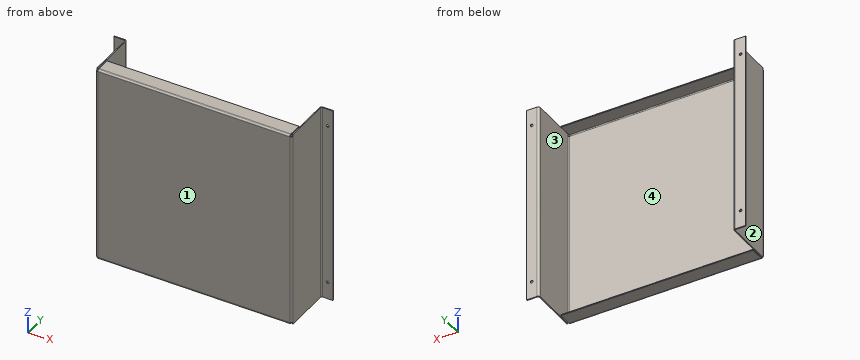
```python
from build123d import *

# Parameters (mm, degrees)
SM_BASE_FLANGE_1_DEPTH   = 200
SM_START                 = -197
SM_EDGE_FLANGE_1_DEPTH   = 394
SM_EDGE_FLANGE_1_2_DEPTH = 4
SM_START_2               = 193
SM_EDGE_FLANGE_1_3_DEPTH = 4
SM_START_3               = -193
SM_EDGE_FLANGE_1_4_DEPTH = 386
SKETCH_12_R              = 2.75
CUT_EXTRUDE_1_DEPTH      = 314.687742827


# Read off the part's stored shape, not the designer's step: Ребро-кромка1
# Sheet-metal steps are written as plain solids
with BuildPart() as part:
    # Sketch 1 → Базовая кромка1 (new, symmetric)
    with BuildSketch(Plane.XY):
        with BuildLine():
            Line((-220, 100), (-199, 100))
            ThreePointArc((-199, 100), (-196.171572875, 98.828427125), (-195, 96))
            Line((-195, 96), (-195, 2))
            ThreePointArc((-195, 2), (-194.414213562, 0.585786438), (-193, 0))
            Line((-193, 0), (193, 0))
            ThreePointArc((193, 0), (194.414213562, 0.585786438), (195, 2))
            Line((195, 2), (195, 96))
            ThreePointArc((195, 96), (196.171572875, 98.828427125), (199, 100))
            Line((199, 100), (220, 100))
            Line((220, 100), (220, 98))
            Line((220, 98), (199, 98))
            ThreePointArc((199, 98), (197.585786438, 97.414213562), (197, 96))
            Line((197, 96), (197, 2))
            ThreePointArc((197, 2), (195.828427125, -0.828427125), (193, -2))
            Line((193, -2), (-193, -2))
            ThreePointArc((-193, -2), (-195.828427125, -0.828427125), (-197, 2))
            Line((-197, 2), (-197, 96))
            ThreePointArc((-197, 96), (-197.585786438, 97.414213562), (-199, 98))
            Line((-199, 98), (-220, 98))
            Line((-220, 98), (-220, 100))
        make_face()
    extrude(amount=SM_BASE_FLANGE_1_DEPTH, both=True)

    # Ребро-кромка1 outline → Ребро-кромка1 (cut)
    with BuildSketch(Plane.YZ.offset(SM_START)):
        with BuildLine():
            ThreePointArc((2, -200), (-0.828427125, -198.828427125), (-2, -196))
            Line((-2, -196), (-2, -200))
            Line((-2, -200), (2, -200))
        make_face()
        with BuildLine():
            ThreePointArc((0, -196), (0.585786438, -197.414213562), (2, -198))
            Line((2, -198), (2, -196))
            Line((2, -196), (0, -196))
        make_face()
        with BuildLine():
            ThreePointArc((2, 198), (0.585786438, 197.414213562), (0, 196))
            Line((0, 196), (2, 196))
            Line((2, 196), (2, 198))
        make_face()
        with BuildLine():
            Line((-2, 200), (-2, 196))
            ThreePointArc((-2, 196), (-0.828427125, 198.828427125), (2, 200))
            Line((2, 200), (-2, 200))
        make_face()
    extrude(amount=SM_EDGE_FLANGE_1_DEPTH, mode=Mode.SUBTRACT)

    # Sm Edge Flange 1 2 outline → Sm Edge Flange 1 2 (cut)
    with BuildSketch(Plane.YZ.offset(SM_START)):
        with BuildLine():
            Line((2, -200), (2, -198))
            ThreePointArc((2, -198), (0.585786438, -197.414213562), (0, -196))
            Line((0, -196), (-2, -196))
            ThreePointArc((-2, -196), (-0.828427125, -198.828427125), (2, -200))
        make_face()
        with BuildLine():
            ThreePointArc((2, 200), (-0.828427125, 198.828427125), (-2, 196))
            Line((-2, 196), (0, 196))
            ThreePointArc((0, 196), (0.585786438, 197.414213562), (2, 198))
            Line((2, 198), (2, 200))
        make_face()
    extrude(amount=SM_EDGE_FLANGE_1_2_DEPTH, mode=Mode.SUBTRACT)

    # Sm Edge Flange 1 3 outline → Sm Edge Flange 1 3 (cut)
    with BuildSketch(Plane.YZ.offset(SM_START_2)):
        with BuildLine():
            Line((2, -200), (2, -198))
            ThreePointArc((2, -198), (0.585786438, -197.414213562), (0, -196))
            Line((0, -196), (-2, -196))
            ThreePointArc((-2, -196), (-0.828427125, -198.828427125), (2, -200))
        make_face()
        with BuildLine():
            ThreePointArc((2, 200), (-0.828427125, 198.828427125), (-2, 196))
            Line((-2, 196), (0, 196))
            ThreePointArc((0, 196), (0.585786438, 197.414213562), (2, 198))
            Line((2, 198), (2, 200))
        make_face()
    extrude(amount=SM_EDGE_FLANGE_1_3_DEPTH, mode=Mode.SUBTRACT)

    # Sm Edge Flange 1 4 outline → Sm Edge Flange 1 4 (add)
    with BuildSketch(Plane.YZ.offset(SM_START_3)):
        with BuildLine():
            ThreePointArc((0, -199.464101616), (0.96472382, -199.863703305), (2, -200))
            Line((2, -200), (29, -200))
            Line((29, -200), (29, -198))
            Line((29, -198), (2, -198))
            ThreePointArc((2, -198), (0.585786438, -197.414213562), (0, -196))
            Line((0, -196), (0, -199.464101616))
        make_face()
        with BuildLine():
            Line((0, 199.464101616), (0, 196))
            ThreePointArc((0, 196), (0.585786438, 197.414213562), (2, 198))
            Line((2, 198), (29, 198))
            Line((29, 198), (29, 200))
            Line((29, 200), (2, 200))
            ThreePointArc((2, 200), (0.96472382, 199.863703305), (0, 199.464101616))
        make_face()
    extrude(amount=SM_EDGE_FLANGE_1_4_DEPTH)

    # Эскиз12 → Вырез-Вытянуть1 (cut, through all)
    with BuildSketch(Plane.XZ.offset(-98)):
        with Locations((210, 165)):
            Circle(SKETCH_12_R)
        with Locations(Location((-210, 165, 0), (0, 0, 180))):
            Circle(SKETCH_12_R)
        with Locations(Location((210, -165, 0), (0, 0, 180))):
            Circle(SKETCH_12_R)
        with Locations((-210, -165)):
            Circle(SKETCH_12_R)
    extrude(amount=-CUT_EXTRUDE_1_DEPTH, mode=Mode.SUBTRACT)


solid = part.part
```
Geometry check sheet. Reference: the model listing, model coordinates, mm. Face numbers are marked on the shaded views. Give positions to 0.01 mm unless a question says otherwise; leave off trailing zeros. Order: outer loops, then holes, each group sorted by start corner. A loop starts at its lowest first (then second) coordinate and runs counter-clockwise, first axis right, second up. Notation, with made-up numbers: (50.25, 78.25) - (102.25, 78.25) arc R26 cw to (102.25, 97.25) - close; hole circle Ø9 at (22, 83). An arc over 180 degrees is marked (long way). Answer in a Markdown table with one row per item. Add a question column.
Q1. Material ranges on probe 1 along Z at (x, y) = (-210, 99); probe 2 along X at (y, z) = (98.6, -165); probe 3 along X at (y, z) = (99.4, -165), recorded low to high. Write a range as from..to.
Q2. Mould release check, pull along X, two halves, no side actions. Record for the marked faces 1, 2, 3 and 4: pulls with the +X half, pulls with the -X half, needs draft (parallel to the pull), parting line crosses it, or undercut.
Q3. Cross-section at B-B, the plane y = 55. Enter the section's corners in (x, z).
Q4. Gauge pin test, flat ends, axial feed: pin 1 (0.6 mm diameter, centred on x = -196, z = -197.5, fed in from -Y); pin 2 (2 mm diameter, centred on x = 196, y = 0.5, fed in from +Z); pin 3 (2 mm diameter, centred on y = 20.5, z = 198.5, fed in from -X). Record the tip position at first contact, or that the pin passes through.
Q5. Cross-section at D-D, the plane z = -24. Enter the section's corners in (x, y), then the cut area to 3 significant figures.
Q6. Cross-section at C-C, the plane x = -186.5. Enter the section's corners in (y, z), then the cut area to 3 significant figures.
Q7. Cross-section at A-A, the plane y = 24. Enter the section's corners in (x, z), then the cut area to 3 significant figures.
Check values:
| question | item | result |
|---|---|---|
| 1 | probe 1 | z = -200..-167.75, -162.25..162.25, 167.75..200 |
| 1 | probe 2 | x = -220..-212.75, -207.25..-195.96, 195.96..207.25, 212.75..220 |
| 1 | probe 3 | x = -220..-212.75, -207.25..-196.89, 196.89..207.25, 212.75..220 |
| 2 | face 1 | needs draft |
| 2 | face 2 | pulls with the -X half |
| 2 | face 3 | undercut |
| 2 | face 4 | undercut |
| 3 | outline | (-197, -200) - (-195, -200) - (-195, 200) - (-197, 200) - close; (195, -200) - (197, -200) - (197, 200) - (195, 200) - close |
| 4 | pin 1 | stops at y = 2 |
| 4 | pin 2 | stops at z = 196 |
| 4 | pin 3 | stops at x = -197 |
| 5 | outline | (-220, 98) - (-199, 98) arc R2 cw to (-197, 96) - (-197, 2) arc R4 ccw to (-193, -2) - (193, -2) arc R4 ccw to (197, 2) - (197, 96) arc R2 cw to (199, 98) - (220, 98) - (220, 100) - (199, 100) arc R4 ccw to (195, 96) - (195, 2) arc R2 cw to (193, 0) - (-193, 0) arc R2 cw to (-195, 2) - (-195, 96) arc R4 ccw to (-199, 100) - (-220, 100) - close |
| 5 | area | 1,270 mm^2 |
| 6 | outline | (-2, -196) arc R4 ccw to (2, -200) - (29, -200) - (29, -198) - (2, -198) arc R2 cw to (0, -196) - (0, 196) arc R2 cw to (2, 198) - (29, 198) - (29, 200) - (2, 200) arc R4 ccw to (-2, 196) - close |
| 6 | area | 911 mm^2 |
| 7 | outline | (-197, -200) - (-195, -200) - (-195, 200) - (-197, 200) - close; (-193, -200) - (193, -200) - (193, -198) - (-193, -198) - close; (-193, 198) - (193, 198) - (193, 200) - (-193, 200) - close; (195, -200) - (197, -200) - (197, 200) - (195, 200) - close |
| 7 | area | 3,140 mm^2 |
